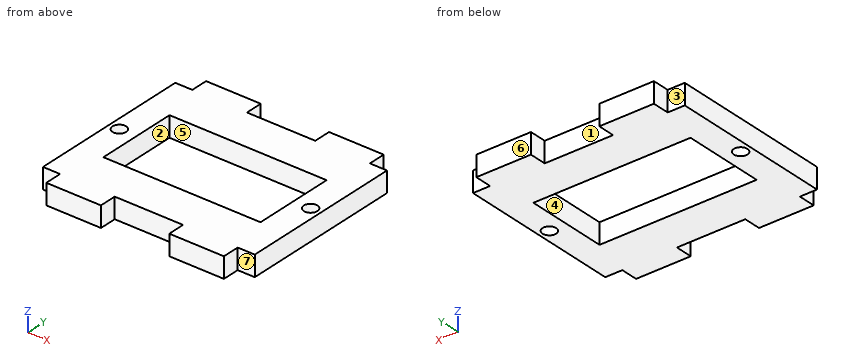
from build123d import *

# Parameters (mm, degrees)
SKETCH1_R           = 1
SKETCH1_W           = 23
SKETCH1_H           = 12
BOSS_EXTRUDE1_DEPTH = 1.5


with BuildPart() as part:
    # Sketch1 → Boss-Extrude1 (new body, symmetric)
    with BuildSketch(Plane.XY):
        Polygon((-13, 12), (-15.5, 12), (-15.5, -12), (-13, -12), (-13, -14.5), (-5, -14.5), (-5, -12), (5, -12), (5, -14.5), (13, -14.5), (13, -12), (15.5, -12), (15.5, 12), (13, 12), (13, 14.5), (5, 14.5), (5, 12), (-5, 12), (-5, 14.5), (-13, 14.5), align=None)
        with Locations((-14, 0)):
            Circle(SKETCH1_R, mode=Mode.SUBTRACT)
        Rectangle(SKETCH1_W, SKETCH1_H, mode=Mode.SUBTRACT)
        with Locations((14, 0)):
            Circle(SKETCH1_R, mode=Mode.SUBTRACT)
    extrude(amount=BOSS_EXTRUDE1_DEPTH, both=True)


solid = part.part
For this review, take the finished solid that the model builds, in its own axes (mm). Face numbers are marked on the shaded views. A direction names the side the tool comes from. Round coordinates to 2 decimals unless told otherwise and drop trailing zeros. Loops run counter-clockwise (first coordinate to the right, second up) from the corner with the lowest first, then second, coordinate; pieces in that order, holes last. Notation, with made-up numbers: (60.5, -33) - (87.5, -33) arc R13 ccw to (87.5, -26) - close; hole circle Ø11 at (51, -34.75). An arc over 180 degrees is marked (long way). One line per item, written item: value. Start each with the question number.
Item 1: Take a section at C-C (z = 0.5). Give the boundary of the cut face in (x, y), plus the area to 3 significant figures.
Item 2: Take a section at A-A (x = -4.5). Give the boundary of the cut face in (y, z).
Item 3: Take a section at B-B (y = 4.25). Give the boundary of the cut face in (x, z), plus the area to 3 significant figures.
Item 4: The part is to be moulded in two halves that separate along Y. For the marked faces 4, 5, 6 and 7, say which applies: +Y half, -Y half, draft (parallel to the pull), parting line (faces both ways), or undercut.
Item 5: For L1, parallel to Y at x = -1, z = 1; L2, parallel to Y at x = -14, z = 0.65; L3, parallel to X at y = 5.25, z = 1.05, list the stretches that pass through material, from the lowest coordinate up.
Item 6: Clearance check with flat-ended pins moving along their axes: pin 1 Ø0.8 at (x, z) = (-14.5, -0.5) entering from -Y; pin 2 Ø0.9 at (x, z) = (-2, -0.5) entering from +Y; pin 3 Ø2.5 at (x, y) = (14, 0) entering from +Z; pin 4 Ø0.8 at (y, z) = (13, 0) entering from -X. State where each tip first meets the part, or that it passes through.
Item 7: For the marked faces 1, 2 and 3, list the 3-axis set-ups (+Z, -Z, +X, -X, +Y, -Y) from which the entire face can be reached by the end or side of a thin tool; tool diameter is ignored.
Item 8: Take a section at D-D (y = 0). Give the boundary of the cut face in (x, z).
Answer below:
1. outline: (-15.5, -12) - (-13, -12) - (-13, -14.5) - (-5, -14.5) - (-5, -12) - (5, -12) - (5, -14.5) - (13, -14.5) - (13, -12) - (15.5, -12) - (15.5, 12) - (13, 12) - (13, 14.5) - (5, 14.5) - (5, 12) - (-5, 12) - (-5, 14.5) - (-13, 14.5) - (-13, 12) - (-15.5, 12) - close; hole circle Ø2 at (-14, 0); hole (-11.5, -6) - (11.5, -6) - (11.5, 6) - (-11.5, 6) - close; hole circle Ø2 at (14, 0)
1. area: 542 mm2
2. outline: (-12, -1.5) - (-6, -1.5) - (-6, 1.5) - (-12, 1.5) - close; (6, -1.5) - (12, -1.5) - (12, 1.5) - (6, 1.5) - close
3. outline: (-15.5, -1.5) - (-11.5, -1.5) - (-11.5, 1.5) - (-15.5, 1.5) - close; (11.5, -1.5) - (15.5, -1.5) - (15.5, 1.5) - (11.5, 1.5) - close
3. area: 24.0 mm2
4. face 4: undercut
4. face 5: undercut
4. face 6: +Y half
4. face 7: -Y half
5. L1: y = -12 to -6, 6 to 12
5. L2: y = -12 to -1, 1 to 12
5. L3: x = -15.5 to -11.5, 11.5 to 15.5
6. pin 1: stops at y = -12
6. pin 2: stops at y = 12
6. pin 3: stops at z = 1.5
6. pin 4: stops at x = -13
7. face 1: +Z, -Z, +Y
7. face 2: +Z, -Z
7. face 3: +Z, -Z, -X, +Y
8. outline: (-15.5, -1.5) - (-15, -1.5) - (-15, 1.5) - (-15.5, 1.5) - close; (-13, -1.5) - (-11.5, -1.5) - (-11.5, 1.5) - (-13, 1.5) - close; (11.5, -1.5) - (13, -1.5) - (13, 1.5) - (11.5, 1.5) - close; (15, -1.5) - (15.5, -1.5) - (15.5, 1.5) - (15, 1.5) - close
